from build123d import *

# Parameters (mm, degrees)
ESQUISSE4_R             = 1.6
ENL_V_MAT_EXTRU_1_DEPTH = 10
ESQUISSE7_W             = 2.232279801
ESQUISSE7_H             = 5
ENL_V_MAT_EXTRU_3_DEPTH = 5


with BuildPart() as part:
    # Esquisse1 → R_volution1 (revolve)
    with BuildSketch(Plane.XY):
        Polygon((0, 30), (-3.196152423, 30), (-4, 33), (-4, 56.025303512), (-2.955946463, 56.025303512), (-2.955946463, 74.525303512), (-1.223895655, 75.525303512), (0, 75.525303512), align=None)
    revolve(axis=Axis((0, 77.095183619, 0), (0, -1, 0)))

    # Esquisse4 → Enl_v. mat.-Extru.1 (cut)
    with BuildSketch(Plane.XZ.offset(-30)):
        with Locations(Location((0, 0, 0), (0, 0, 270))):
            Circle(ESQUISSE4_R)
    extrude(amount=-ENL_V_MAT_EXTRU_1_DEPTH, mode=Mode.SUBTRACT)

    # Esquisse7 → Enl_v. mat.-Extru.3 (cut, symmetric)
    with BuildSketch(Plane(origin=(0, 0, 0), x_dir=(0, 0, -1), z_dir=(1, 0, 0))):
        with Locations((-3.116139901, 63.525303512)):
            Rectangle(ESQUISSE7_W, ESQUISSE7_H)
        with Locations((3.116139901, 63.525303512)):
            Rectangle(ESQUISSE7_W, ESQUISSE7_H)
    extrude(amount=ENL_V_MAT_EXTRU_3_DEPTH, both=True, mode=Mode.SUBTRACT)


solid = part.part
CAD build for the part. Positions are in the model's coordinates, mm. A direction names the side the tool comes from. Give positions to 0.01 mm unless a question says otherwise; leave off trailing zeros. Write each loop counter-clockwise with the first axis right and the second up, starting at its lowest first coordinate (ties: lowest second). Pieces come first, ordered by that corner, then holes. Notation, with made-up numbers: (-6, 46.25) -> (10, 46.25) arc R18 ccw to (10, 52.25) -> close; hole circle Ø2 at (70.5, -21.75). An arc over 180 degrees is marked (long way). Return JSON: item names as keys, results as strings.
Item 1: Drop flat-ended pins along their axis: pin 1 (2 mm diameter, centred on x = 1, y = 62.5, fed in from +Z); pin 2 (1.3 mm diameter, centred on x = -0.5, y = 64.5, fed in from -Z); pin 3 (4 mm diameter, centred on x = -3, y = 50, fed in from +Z). Give the stop position or say it passes through.
Answer below:
{"pin 1": "stops at z = 2", "pin 2": "stops at z = -2", "pin 3": "stops at z = 3.87"}
Item 2: Band-saw the part on A-A (x = 0). List the corners of the cut face in (y, z).
Answer below:
{"outline": "(30, -3.2) -> (33, -4) -> (56.03, -4) -> (56.03, -2.96) -> (61.03, -2.96) -> (61.03, -2) -> (66.03, -2) -> (66.03, -2.96) -> (74.53, -2.96) -> (75.53, -1.22) -> (75.53, 1.22) -> (74.53, 2.96) -> (66.03, 2.96) -> (66.03, 2) -> (61.03, 2) -> (61.03, 2.96) -> (56.03, 2.96) -> (56.03, 4) -> (33, 4) -> (30, 3.2) -> (30, 1.6) -> (40, 1.6) -> (40, -1.6) -> (30, -1.6) -> close"}
Item 3: Drill centre lines: probe 1 along X at (y, z) = (37.5, 0); probe 2 along Z at (x, y) = (-2, 63); probe 3 along Z at (x, y) = (0.5, 33). Where is each one in solid material? Low to high.
Answer below:
{"probe 1": "x = -4 to -1.6, 1.6 to 4", "probe 2": "z = -2 to 2", "probe 3": "z = -3.97 to -1.52, 1.52 to 3.97"}
Item 4: Two-plate mould, pull along X, no slides. Class faces 1 (the cylindrical face through (0.867, 44.674, 3.905)), 2 (the flat face through (0, 40, 0)), 3 (the flat face through (0, 75.525, 0)): +X half, -X half, draft (parallel to the pull), parting line (faces both ways), or undercut.
Answer below:
{"face 1": "parting line", "face 2": "undercut", "face 3": "draft"}
Item 5: Band-saw the part on B-B (z = 0). List the corners of the cut face in (x, y), then the cut area to 3 significant figures.
Answer below:
{"outline": "(-4, 33) -> (-3.2, 30) -> (-1.6, 30) -> (-1.6, 40) -> (1.6, 40) -> (1.6, 30) -> (3.2, 30) -> (4, 33) -> (4, 56.03) -> (2.96, 56.03) -> (2.96, 74.53) -> (1.22, 75.53) -> (-1.22, 75.53) -> (-2.96, 74.53) -> (-2.96, 56.03) -> (-4, 56.03) -> close", "area": "287 mm2"}
Item 6: Band-saw the part on D-D (y = 63.5). List the corners of the cut face in (x, z).
Answer below:
{"outline": "(-2.18, -2) -> (2.18, -2) arc R2.96 ccw to (2.18, 2) -> (-2.18, 2) arc R2.96 ccw to start"}
Item 7: Band-saw the part on C-C (y = 51). List the corners of the cut face in (x, z), then the cut area to 3 significant figures.
Answer below:
{"outline": "circle Ø8 at (0, 0)", "area": "50.3 mm2"}
Item 8: Tool access for faces 4 (the flat face through (0, 66.025, 2.4)), 5 (the flat face through (0, 61.025, -2.4)), 6 (the cylindrical face through (2.953, 65.405, -0.13)), 7 (the cylindrical face through (-0.97, 34.93, 1.27)): list every direction of +Z, -Z, +X, -X, +Y, -Y with a clear straight run to the whole face (end or side of a thin tool).
Answer below:
{"face 4": "+Z, +X, -X", "face 5": "-Z, +X, -X", "face 6": "+Y", "face 7": "-Y"}
